Part print with two shaded views. Sizes in mm from the minimum x, y, z corner. A direction names the side the tool comes from. Round coordinates to 2 decimals unless told otherwise and drop trailing zeros. Order: outer loops, then holes, each group sorted by start corner. A loop starts at its lowest first (then second) coordinate and runs counter-clockwise, first axis right, second up. Notation, with made-up numbers: (25.5, -40) - (62.5, -40) arc R15 ccw to (62.5, -21) - close; hole circle Ø9 at (67.25, 59). An arc over 180 degrees is marked (long way). Use one line per item in the form item = value.
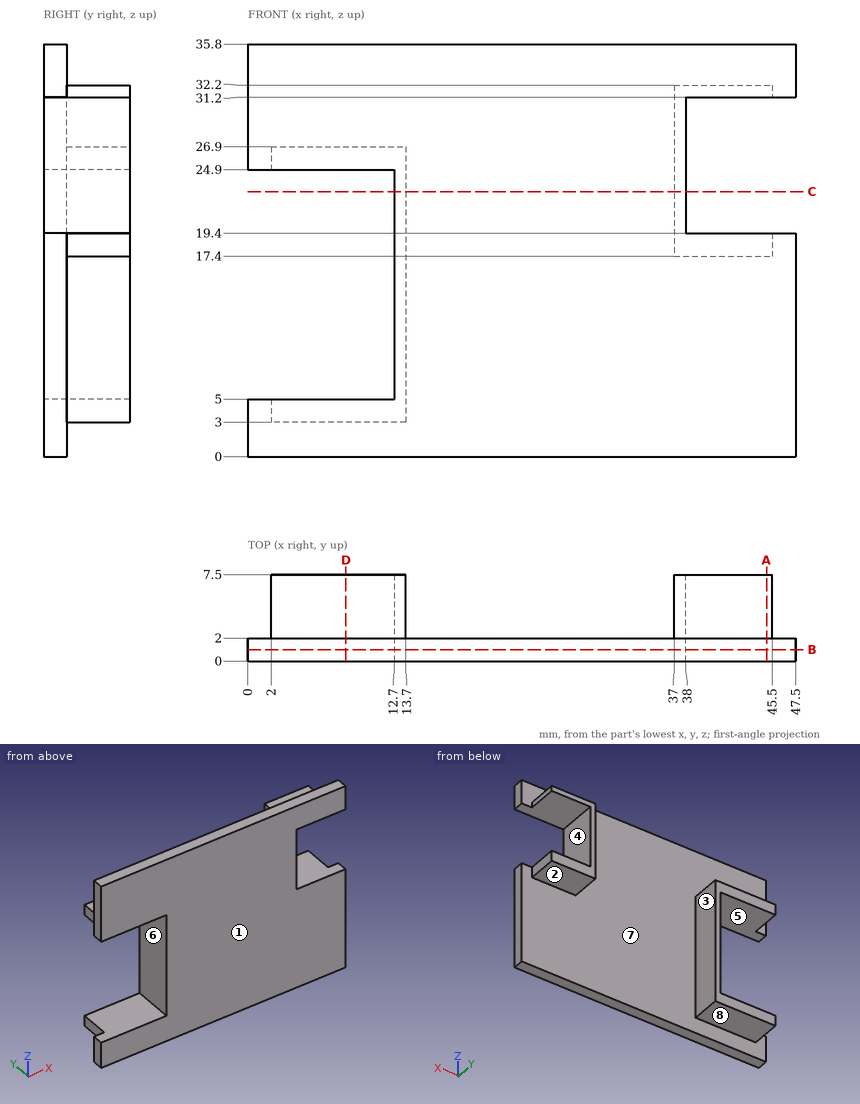
(1) Slice it at D-D on x = 8.5. Give the cut face in (y, z).
Report:
outline = (0, 0) - (2, 0) - (2, 3) - (7.5, 3) - (7.5, 5) - (0, 5) - close; (0, 24.9) - (7.5, 24.9) - (7.5, 26.9) - (2, 26.9) - (2, 35.8) - (0, 35.8) - close
(2) Tool access for the marked faces 1, 2, 3, 4 and 5: list every direction of +Z, -Z, +X, -X, +Y, -Y with a clear straight run to the whole face (end or side of a thin tool).
Report:
face_1 = +Z, -Z, +X, -X, -Y
face_2 = -Z, +X, +Y
face_3 = +Z, -Z, +Y
face_4 = +X, +Y, -Y
face_5 = -X, +Y, -Y
(3) Pin check, flat tips, straight feed: pin 1 (0.8 mm diameter, centred on y = 4, z = 32, fed in from +X); pin 2 (4.5 mm diameter, centred on x = 9, y = 6, fed in from +Z); pin 3 (3 mm diameter, centred on y = 1, z = 23.5, fed in from +X). Stop position of each tip, or through.
Report:
pin_1 = 45.5
pin_2 = 26.9
pin_3 = 38
(4) Slice it at C-C on z = 23. Give the cut face in (x, y), then the cut area to 3 significant figures.
Report:
outline = (12.7, 0) - (38, 0) - (38, 7.5) - (37, 7.5) - (37, 2) - (13.7, 2) - (13.7, 7.5) - (12.7, 7.5) - close
area = 61.6 mm2
(5) Slice it at B-B on y = 1. Give the cut face in (x, z).
Report:
outline = (0, 0) - (47.5, 0) - (47.5, 19.4) - (38, 19.4) - (38, 31.2) - (47.5, 31.2) - (47.5, 35.8) - (0, 35.8) - (0, 24.9) - (12.7, 24.9) - (12.7, 5) - (0, 5) - close
(6) Pull direction Z, two halves, no side cores. Call the marked faces 6, 7 and 8: released by +Z, released by -Z, zero draft, split by the parting line, or undercut.
Report:
face_6 = undercut
face_7 = zero draft
face_8 = released by -Z
(7) Probe probe 1 along Z at (x, y) = (42.5, 1); probe 2 along X at (y, z) = (3.75, 18); probe 3 along X at (y, z) = (3.75, 26). List the from-to ranges inside material, lowest first. Write a range as [from, to].
Report:
probe_1 = [0, 19.4], [31.2, 35.8]
probe_2 = [12.7, 13.7], [37, 45.5]
probe_3 = [2, 13.7], [37, 38]
(8) Slice it at A-A on x = 45. Give the cut face in (y, z).
Report:
outline = (0, 0) - (2, 0) - (2, 17.4) - (7.5, 17.4) - (7.5, 19.4) - (0, 19.4) - close; (0, 31.2) - (7.5, 31.2) - (7.5, 32.2) - (2, 32.2) - (2, 35.8) - (0, 35.8) - close
